Could you check a few things on this model? Use its own coordinates, in mm. Round coordinates to 2 decimals unless told otherwise and drop trailing zeros. Write each loop counter-clockwise with the first axis right and the second up, starting at its lowest first coordinate (ties: lowest second). Pieces come first, ordered by that corner, then holes. Notation, with made-up numbers: (38, 50) -> (74, 50) arc R9 cw to (74, 65) -> close; hole circle Ø5 at (6, 60.5). An arc over 180 degrees is marked (long way). One line per question, with ' | ' between items. Start each with the question number.
1. For pin 1 Ø0.6 at (x, z) = (-79.5, 52) entering from -Y; pin 2 Ø6 at (y, z) = (-44.5, 50.5) entering from -X; pin 3 Ø2 at (x, z) = (-97, 41) entering from -Y; pin 4 Ø0.6 at (x, z) = (-90.5, 49.5) entering from +Y, each with a flat end and sliding along its axis, tell me the tip position at first contact or that it passes through.
2. Imagine slicing it at C-C, the plane z = 38.75. List the corners of the cut face in (x, y) for me, and give its area (3 significant figures).
3. Imagine slicing it at D-D, the plane y = -26. List the corners of the cut face in (x, z) for me, and give its area (3 significant figures).
4. Imagine slicing it at B-B, the plane x = -69.5. List the corners of the cut face in (y, z) for me.
5. If I drill on line 1 along Y through (x, z) = (-84.5, 43.25); line 2 along Y through (x, z) = (-81, 58.75); line 3 along Y through (x, z) = (-66, 48.5), over which ranges is the centre line in solid material (lowest first)? Write a range as [from, to].
6. Thinking about a two-plate mould opening in Y: for faces 1 (the cylindrical face through (-89.647, -65.036, 49.456)), 2 (the flat face through (-84, -43, 35.8)), 3 (the cylindrical face through (-79.63, -38.17, 54.16)), 4 (the cylindrical face through (-80.95, -46.29, 54.16)), which applies, released by +Y, released by -Y, zero draft, split by the parting line, or undercut?
from build123d import *

# Parameters (mm, degrees)
SKETCH1_W                      = 22.51077
SKETCH1_H                      = 27.7
CUT_EXTRUDE1_DEPTH             = 18.95
F_7_5_7_5_DIAMETER_HOLE1_D     = 7.5
F_7_5_7_5_DIAMETER_HOLE1_DEPTH = 3.75


with BuildPart() as part:
    # Sketch1 → Revolve1 (revolve)
    with BuildSketch(Plane(origin=(0, -43.060148556, 0), x_dir=(1, 0, 0), z_dir=(0, 1, 0))):
        with Locations((-73.512097724, -49.65)):
            Rectangle(SKETCH1_W, SKETCH1_H)
    revolve(axis=Axis((-84.767482724, -43.060148556, 35.8), (0, 0, 1)))

    # Sketch2 → Cut-Extrude1 (cut)
    with BuildSketch(Plane.XY.offset(63.5)):
        with BuildLine():
            Line((-85.635723612, -38.136109791), (-85.830856299, -37.029457332))
            ThreePointArc((-85.830856299, -37.029457332), (-86.451441226, -36.155700609), (-87.520742643, -36.083791354))
            ThreePointArc((-87.520742643, -36.083791354), (-87.997695155, -36.833554149), (-87.855939444, -37.7107846))
            Line((-87.855939444, -37.7107846), (-87.267482724, -38.730021537))
            ThreePointArc((-87.267482724, -38.730021537), (-88.597704939, -39.846210508), (-89.465945828, -41.350047839))
            Line((-89.465945828, -41.350047839), (-90.521901314, -40.965711474))
            ThreePointArc((-90.521901314, -40.965711474), (-91.588889296, -41.066275425), (-92.185815247, -41.956362989))
            ThreePointArc((-92.185815247, -41.956362989), (-91.774977875, -42.744297377), (-90.944396164, -43.060148556))
            Line((-90.944396164, -43.060148556), (-89.767482724, -43.060148556))
            ThreePointArc((-89.767482724, -43.060148556), (-89.465945828, -44.770249273), (-88.597704939, -46.274086605))
            Line((-88.597704939, -46.274086605), (-89.458527739, -46.996402698))
            ThreePointArc((-89.458527739, -46.996402698), (-89.904930794, -47.970723371), (-89.432555327, -48.932720191))
            ThreePointArc((-89.432555327, -48.932720191), (-88.544765444, -48.970891785), (-87.855939444, -48.409512512))
            Line((-87.855939444, -48.409512512), (-87.267482724, -47.390275575))
            ThreePointArc((-87.267482724, -47.390275575), (-85.635723612, -47.984187321), (-83.899241835, -47.984187321))
            Line((-83.899241835, -47.984187321), (-83.704109149, -49.09083978))
            ThreePointArc((-83.704109149, -49.09083978), (-83.083524222, -49.964596503), (-82.014222804, -50.036505758))
            ThreePointArc((-82.014222804, -50.036505758), (-81.537270293, -49.286742964), (-81.679026004, -48.409512512))
            Line((-81.679026004, -48.409512512), (-82.267482724, -47.390275575))
            ThreePointArc((-82.267482724, -47.390275575), (-80.937260508, -46.274086605), (-80.06901962, -44.770249273))
            Line((-80.06901962, -44.770249273), (-79.013064134, -45.154585638))
            ThreePointArc((-79.013064134, -45.154585638), (-77.946076152, -45.054021688), (-77.349150201, -44.163934124))
            ThreePointArc((-77.349150201, -44.163934124), (-77.759987572, -43.375999735), (-78.590569284, -43.060148556))
            Line((-78.590569284, -43.060148556), (-79.767482724, -43.060148556))
            ThreePointArc((-79.767482724, -43.060148556), (-80.06901962, -41.350047839), (-80.937260508, -39.846210508))
            Line((-80.937260508, -39.846210508), (-80.076437709, -39.123894414))
            ThreePointArc((-80.076437709, -39.123894414), (-79.630034654, -38.149573741), (-80.10241012, -37.187576921))
            ThreePointArc((-80.10241012, -37.187576921), (-80.990200003, -37.149405327), (-81.679026004, -37.7107846))
            Line((-81.679026004, -37.7107846), (-82.267482724, -38.730021537))
            ThreePointArc((-82.267482724, -38.730021537), (-83.899241835, -38.136109791), (-85.635723612, -38.136109791))
        make_face()
    extrude(amount=-CUT_EXTRUDE1_DEPTH, mode=Mode.SUBTRACT)

    # Ø7.5 (7.5) Diameter Hole1
    with Locations(Plane.XY.offset(44.55)):
        with Locations((-84.767482724, -43.060148556)):
            Hole(F_7_5_7_5_DIAMETER_HOLE1_D / 2, depth=F_7_5_7_5_DIAMETER_HOLE1_DEPTH)


solid = part.part
Geometry results:
1) pin 1: stops at y = -65.02 | pin 2: stops at x = -107.28 | pin 3: stops at y = -62.57 | pin 4: stops at y = -21.21
2) outline: circle Ø45.02 at (-84.77, -43.06) | area: 1,590 mm2
3) outline: (-99.45, 35.8) -> (-70.08, 35.8) -> (-70.08, 63.5) -> (-99.45, 63.5) -> close | area: 814 mm2
4) outline: (-59.6, 35.8) -> (-26.52, 35.8) -> (-26.52, 63.5) -> (-59.6, 63.5) -> close
5) line 1: y = [-65.57, -46.8], [-39.32, -20.55] | line 2: y = [-65.25, -46.35], [-37.15, -20.87] | line 3: y = [-55.49, -30.63]
6) face 1: split by the parting line | face 2: zero draft | face 3: undercut | face 4: undercut
